```python
from build123d import *

# Parameters (mm, degrees)
SKETCH1_R           = 1.75
BOSS_EXTRUDE1_DEPTH = 8.5
CUT_EXTRUDE2_DEPTH  = 2.5
CUT_EXTRUDE3_DEPTH  = 2.5
SKETCH5_R           = 3.5
CUT_EXTRUDE4_DEPTH  = 3.5
SKETCH6_R           = 3.5
CUT_EXTRUDE5_DEPTH  = 3.5
FILLET1_R           = 11.4
SKETCH7_W           = 8.501662988
SKETCH7_H           = 41.75
BOSS_EXTRUDE3_DEPTH = 8.5
SKETCH8_W           = 5
SKETCH8_H           = 28.902484154
CUT_EXTRUDE6_DEPTH  = 44.858046851
CUT_EXTRUDE7_REACH  = 52.235
FILLET2_R           = 5
FILLET3_R           = 5


with BuildPart() as part:
    # Sketch1 → Boss-Extrude1 (new body)
    with BuildSketch(Plane.XY):
        Polygon((8, -10), (8, -27), (-25, -27), (-25, 14.75), align=None)
        with Locations((-20, 1)):
            Circle(SKETCH1_R, mode=Mode.SUBTRACT)
        with Locations((0, -14)):
            Circle(SKETCH1_R, mode=Mode.SUBTRACT)
        Polygon((-6.687894354, -19), (-6.666666667, -19), (-6.687894354, -18.984079234), align=None, mode=Mode.SUBTRACT)
    extrude(amount=BOSS_EXTRUDE1_DEPTH)

    # Sketch3 → Cut-Extrude2 (cut)
    with BuildSketch(Plane(origin=(0, 0, 0), x_dir=(-1, 0, 0), z_dir=(0, 0, -1))):
        Polygon((22.725, 2.573279484), (20, 4.146558967), (17.275, 2.573279484), (17.275, -0.573279484), (20, -2.146558967), (22.725, -0.573279484), align=None)
    extrude(amount=-CUT_EXTRUDE2_DEPTH, mode=Mode.SUBTRACT)

    # Sketch4 → Cut-Extrude3 (cut)
    with BuildSketch(Plane.XY.offset(8.5)):
        Polygon((-2.517247174, -12.11206462), (-2.893623587, -15.23603231), (-0.376376413, -17.12396769), (2.517247174, -15.88793538), (2.893623587, -12.76396769), (0.376376413, -10.87603231), align=None)
    extrude(amount=-CUT_EXTRUDE3_DEPTH, mode=Mode.SUBTRACT)

    # Sketch5 → Cut-Extrude4 (cut)
    with BuildSketch(Plane.XY.offset(8.5)):
        with Locations((-20, 1)):
            Circle(SKETCH5_R)
    extrude(amount=-CUT_EXTRUDE4_DEPTH, mode=Mode.SUBTRACT)

    # Sketch6 → Cut-Extrude5 (cut)
    with BuildSketch(Plane(origin=(0, 0, 0), x_dir=(-1, 0, 0), z_dir=(0, 0, -1))):
        with Locations((0, -14)):
            Circle(SKETCH6_R)
    extrude(amount=-CUT_EXTRUDE5_DEPTH, mode=Mode.SUBTRACT)

    # Fillet1
    # the kernel refuses this fillet: 11.4 mm, written as the material it takes off along each edge
    with BuildSketch(Plane(origin=(8, -10, -14.25), x_dir=(0, -1, 0), z_dir=(0, 0, 1))) as fillet1_piece_1:
        with BuildLine():
            CenterArc((FILLET1_R * 0.5, -FILLET1_R), FILLET1_R, 90, 53.130102354)
            Line((-FILLET1_R * 0.3, -FILLET1_R * 0.4), (0, 0))
            Line((0, 0), (FILLET1_R * 0.5, 0))
        make_face()
    extrude(amount=37, mode=Mode.SUBTRACT)
    with BuildSketch(Plane(origin=(8, -27, -28.5), x_dir=(0, 1, 0), z_dir=(0, 0, 1))) as fillet1_piece_2:
        with BuildLine():
            CenterArc((FILLET1_R, FILLET1_R), FILLET1_R, 180, 90)
            Line((0, FILLET1_R), (0, 0))
            Line((0, 0), (FILLET1_R, 0))
        make_face()
    extrude(amount=65.5, mode=Mode.SUBTRACT)

    # Sketch7 → Boss-Extrude3 (add)
    with BuildSketch(Plane.ZY.offset(25)):
        with Locations((4.25, -6.125)):
            Rectangle(SKETCH7_W, SKETCH7_H)
    extrude(amount=BOSS_EXTRUDE3_DEPTH)

    # Sketch8 → Cut-Extrude6 (cut, through all)
    with BuildSketch(Plane.XY.offset(8.500831494)):
        with Locations((-27.983222081, -5.565864812)):
            Rectangle(SKETCH8_W, SKETCH8_H)
    extrude(amount=-CUT_EXTRUDE6_DEPTH, mode=Mode.SUBTRACT)

    # Sketch9 → Cut-Extrude7 (cut, up to next)
    with BuildSketch(Plane.ZY.offset(33.5), mode=Mode.PRIVATE) as cut_extrude7_sk1:
        with BuildLine():
            Line((5.75, -17.038286927), (5.75, 5.275984322))
            ThreePointArc((5.75, 5.275984322), (4.25, 6.775984322), (2.75, 5.275984322))
            Line((2.75, 5.275984322), (2.75, -17.038286927))
            ThreePointArc((2.75, -17.038286927), (4.25, -18.194874392), (5.75, -17.038286927))
        make_face()
    cut_extrude7_tool1 = extrude(cut_extrude7_sk1.sketch, amount=-CUT_EXTRUDE7_REACH, mode=Mode.PRIVATE) & part.part
    add(cut_extrude7_tool1.solids().sort_by_distance((-33.5, -5.719772, 4.25))[0], mode=Mode.SUBTRACT)

    # Fillet2
    fillet2_edges = [part.edges().sort_by_distance(p)[0] for p in [
        (-33.5, -27, 4.25),
    ]]
    fillet(fillet2_edges, radius=FILLET2_R)

    # Fillet3
    fillet3_edges = [part.edges().sort_by_distance(p)[0] for p in [
        (-33.5, 14.75, 4.25),
    ]]
    fillet(fillet3_edges, radius=FILLET3_R)


solid = part.part
```
Part model, mm, in its own coordinate system. A direction names the side the tool comes from. Round coordinates to 2 decimals unless told otherwise and drop trailing zeros.
Item 1: Drill centre lines: line 1 (X direction, y = -4, z = 0.5); line 2 (X direction, y = 1, z = 4.2); line 3 (Y direction, x = -28.5, z = 2.5). Where is each one in solid material? Low to high.
Item 2: 3-axis set-ups, long thin cutter, end or side, ignore diameter. For faces 5 (the face through (-21.343, -1.371, 1.232)), 6 (the face through (-30.483, -6, 6)), 7 (the face through (-1.65, -16.17, 7.27)): which of +Z, -Z, +X, -X, +Y, -Y reach the whole face in a straight line?
Item 3: Cut at A-A, the plane y = 1. State how many separate pieces and enclosed holes the cut face has, then the cut area to 3 significant figures.
Item 4: Mould opens along Y. For faces 1 (the face through (-32.07, 13.25, 4.31)), 2 (the face through (-31, -6, 8.501)), 3 (the face through (-16.66, 2.05, 6.77)), 4 (the face through (1.05, -16.515, 7.268)) say: +Y half, -Y half, draft (parallel to the pull), parting line (faces both ways), or undercut.
Item 5: Drop flat-ended pins along their axis: P1, Ø5, axis at y = -5.5, z = 4, coming from the +X side; P2, Ø1.5, axis at y = 4, z = 3, coming from the +X side; P3, Ø2, axis at y = 0.5, z = 1.5, coming from the +X side. Give the stop position or say it passes through.
A:
1. line 1: x = -33.5 to -30.48, -25.48 to 0
1. line 2: x = -25.48 to -21.75, -18.25 to -6.67
1. line 3: y = -27 to -20.02, 8.89 to 14.75
2. face 5: -Z
2. face 6: +Z, -Z
2. face 7: +Z
3. separate pieces: 4
3. enclosed holes: 0
3. area: 130 mm2
4. face 1: +Y half
4. face 2: draft
4. face 3: undercut
4. face 4: undercut
5. P1: stops at x = 5.01
5. P2: stops at x = -9.67
5. P3: stops at x = -4.67
